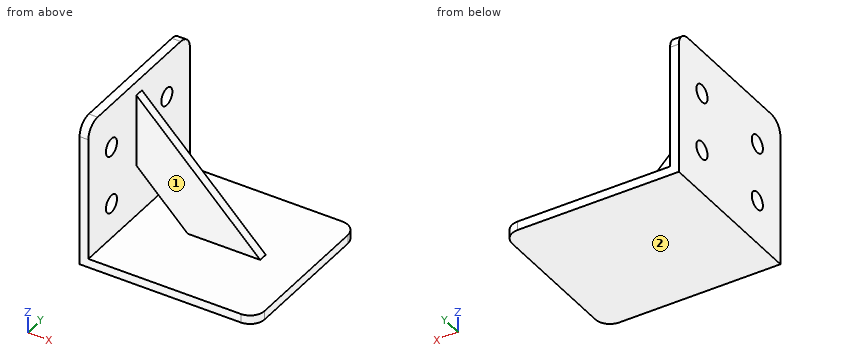
from build123d import *

# Parameters (mm, degrees)
F1_DEPTH = 55
F2_DEPTH = 3
F3_R     = 6
F4_DEPTH = 120.001
F5_R     = 10


with BuildPart() as f1:
    # F0 (on Front) → F1 (new body, symmetric)
    with BuildSketch(Plane.XZ):
        Polygon((0, 100), (0, 0), (120, 0), (120, 6), (90.497475, 6), (41, 6), (6, 6), (6, 41), (6, 90.497475), (6, 100), align=None)
    extrude(amount=F1_DEPTH, both=True)

    # F0 (on Front) → F2 (join, symmetric)
    with BuildSketch(Plane.XZ):
        Polygon((41, 6), (90.497475, 6), (6, 90.497475), (6, 41), align=None)
    extrude(amount=F2_DEPTH, both=True)

    # F3 (on face) → F4 (cut, through all)
    with BuildSketch(Plane(origin=(0, 0, 0), x_dir=(0, -1, 0), z_dir=(-1, 0, 0))):
        with Locations((-30, 70)):
            Circle(F3_R)
        with Locations((30, 70)):
            Circle(F3_R)
        with Locations((30, 30)):
            Circle(F3_R)
        with Locations((-30, 30)):
            Circle(F3_R)
    extrude(amount=-F4_DEPTH, mode=Mode.SUBTRACT)

    # F5
    f5_edges = [f1.edges().sort_by_distance(p)[0] for p in [
        (3, -55, 100),
        (120, -55, 3),
        (120, 55, 3),
        (3, 55, 100),
    ]]
    fillet(f5_edges, radius=F5_R)


solid = f1.part
Work out the finished part from the listing and answer in its coordinate system (mm). Face numbers are marked on the shaded views. A direction names the side the tool comes from. Round coordinates to 2 decimals unless told otherwise and drop trailing zeros. Write each loop counter-clockwise with the first axis right and the second up, starting at its lowest first coordinate (ties: lowest second). Pieces come first, ordered by that corner, then holes. Notation, with made-up numbers: (-1.5, -10.5) -> (57.5, -10.5) arc R22 cw to (57.5, 13.5) -> close; hole circle Ø4 at (64.5, 28.25). An arc over 180 degrees is marked (long way). Answer as CSV lines item,"result". Start each with the question number.
(1) Find the intervals of material crossed by probe 1 along Z at (x, y) = (3.5, 30); probe 2 along Y at (x, z) = (13, 65); probe 3 along X at (y, z) = (9.5, 58.5), in increasing order.
(2) The part is cut by section C-C, the plane z = 30. Give the vertices of the cut face in (x, y), then the cut area to 3 significant figures.
(3) The part is cut by section D-D, the plane z = 67. Give the vertices of the cut face in (x, y), then the cut area to 3 significant figures.
(4) The part is cut by section A-A, the plane y = -30. Give the vertices of the cut face in (x, z), then the cut area to 3 significant figures.
(5) A tool of negligible diameter and unlimited length cuts with its end or side. For the marked faces 1 and 2, from which of +Z, -Z, +X, -X, +Y, -Y can it reach the whole face along a straight path? Write none if from no direction.
(6) The part is cut by section B-B, the plane x = 13. Give the vertices of the cut face in (y, z), then the cut area to 3 significant figures.
(7) Each of these flat-tipped pins is pushed along its axis until it touches: pin 1 (1 mm diameter, centred on y = 3, z = 26, fed in from +X); pin 2 (5 mm diameter, centred on y = -21, z = 36.5, fed in from +X); pin 3 (9.5 mm diameter, centred on y = 30, z = 70, fed in from +X); pin 4 (3 mm diameter, centred on x = 28.5, z = 17.5, fed in from -Y). Where does it stop, or does it pass through?
Output values:
1,probe 1,"z = 0 to 24, 36 to 64, 76 to 100"
1,probe 2,"y = -3 to 3"
1,probe 3,"x = 0 to 6"
2,outline,"(0, -55) -> (6, -55) -> (6, -36) -> (0, -36) -> close; (0, -24) -> (6, -24) -> (6, 24) -> (0, 24) -> close; (0, 36) -> (6, 36) -> (6, 55) -> (0, 55) -> close; (17, -3) -> (66.5, -3) -> (66.5, 3) -> (17, 3) -> close"
2,area,"813 mm²"
3,outline,"(0, -55) -> (6, -55) -> (6, -35.2) -> (0, -35.2) -> close; (0, -24.8) -> (6, -24.8) -> (6, -3) -> (29.5, -3) -> (29.5, 3) -> (6, 3) -> (6, 24.8) -> (0, 24.8) -> close; (0, 35.2) -> (6, 35.2) -> (6, 55) -> (0, 55) -> close"
3,area,"676 mm²"
4,outline,"(0, 0) -> (120, 0) -> (120, 6) -> (6, 6) -> (6, 24) -> (0, 24) -> close; (0, 36) -> (6, 36) -> (6, 64) -> (0, 64) -> close; (0, 76) -> (6, 76) -> (6, 100) -> (0, 100) -> close"
4,area,"1,140 mm²"
5,face 1,"+Z, +X, -Y"
5,face 2,"-Z, +X, -X, +Y, -Y"
6,outline,"(-55, 0) -> (55, 0) -> (55, 6) -> (-55, 6) -> close; (-3, 34) -> (3, 34) -> (3, 83.5) -> (-3, 83.5) -> close"
6,area,"957 mm²"
7,pin 1,"stops at x = 71"
7,pin 2,"stops at x = 6"
7,pin 3,"passes through"
7,pin 4,"stops at y = -3"
